Design review of the part built by this model. Coordinates are the model's own, in mm. Face numbers are marked on the shaded views. A direction names the side the tool comes from. Coordinates: 2 decimals unless noted, no trailing zeros. Loops run counter-clockwise (first coordinate to the right, second up) from the corner with the lowest first, then second, coordinate; pieces in that order, holes last. Notation, with made-up numbers: (73.25, -13) - (127.25, -13) arc R14 cw to (127.25, 9) - close; hole circle Ø7 at (6, 73). An arc over 180 degrees is marked (long way). Return JSON: item names as keys, results as strings. Group by question number.
from build123d import *

# Parameters (mm, degrees)
BOSS_EXTRUDE1_DEPTH         = 41.5925
SHELL1_START                = -39.0525
SHELL1_DEPTH                = 78.105
BOSS_EXTRUDE2_START         = 38.1
SKETCH3_R                   = 12.7
BOSS_EXTRUDE2_DEPTH         = 38.1
SKETCH4_R                   = 11.43
CUT_EXTRUDE1_DEPTH          = 132.301928586
F_1_4_20_TAPPED_HOLE1_D     = 5.1054
F_1_4_20_TAPPED_HOLE1_DEPTH = 2.54


# Read off the part's stored shape, not the designer's step: Shell1
with BuildPart() as part:
    # Sketch2 → Boss-Extrude1 (new, symmetric)
    with BuildSketch(Plane.XY):
        with BuildLine():
            Line((9.525, 8.400260413), (28.575, 41.395828297))
            Line((28.575, 41.395828297), (-28.575, 41.395828297))
            Line((-28.575, 41.395828297), (-9.525, 8.400260413))
            ThreePointArc((-9.525, 8.400260413), (0, -12.7), (9.525, 8.400260413))
        make_face()
    extrude(amount=BOSS_EXTRUDE1_DEPTH, both=True)

    # Shell1 outline → Shell1 (cut)
    with BuildSketch(Plane.XY.offset(SHELL1_START)):
        with BuildLine():
            ThreePointArc((-6.330300915, 7.946879282), (0, -10.16), (6.330300915, 7.946879282))
            Line((6.330300915, 7.946879282), (25.642060633, 41.395828297))
            Line((25.642060633, 41.395828297), (-25.642060633, 41.395828297))
            Line((-25.642060633, 41.395828297), (-6.330300915, 7.946879282))
        make_face()
    extrude(amount=SHELL1_DEPTH, mode=Mode.SUBTRACT)

    # Sketch3 → Boss-Extrude2 (add)
    with BuildSketch(Plane.XY.offset(41.5925).offset(BOSS_EXTRUDE2_START)):
        with Locations(Location((0, 0, 0), (0, 0, 138.590377891))):
            Circle(SKETCH3_R)
    extrude(amount=-BOSS_EXTRUDE2_DEPTH)

    # Sketch4 → Cut-Extrude1 (cut, through all)
    with BuildSketch(Plane.XY.offset(79.6925)):
        Circle(SKETCH4_R)
    extrude(amount=-CUT_EXTRUDE1_DEPTH, mode=Mode.SUBTRACT)

    # 1/4-20 Tapped Hole1
    with Locations(Plane(origin=(0, 0, -41.5925), x_dir=(1, 0, 0), z_dir=(0, 0, -1))):
        with Locations((0, -35.045828297)):
            Hole(F_1_4_20_TAPPED_HOLE1_D / 2, depth=F_1_4_20_TAPPED_HOLE1_DEPTH)


solid = part.part
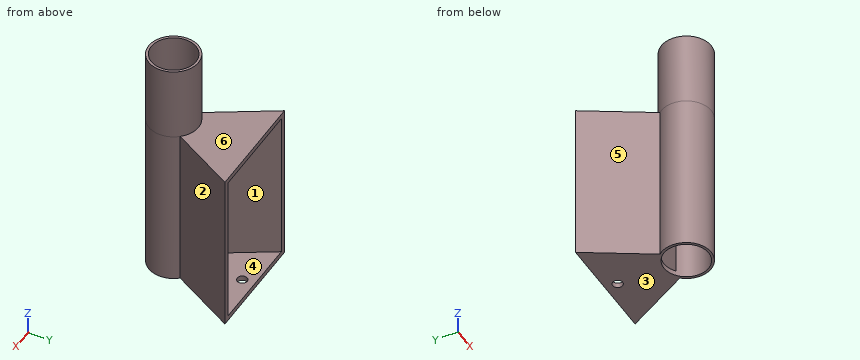
Item 1: Add section D-D (y = 20.5). State the section outline as (x, z) points, then the cut area to 3 significant figures.
Item 2: For the marked faces 1, 2 and 3, list the 3-axis set-ups (+Z, -Z, +X, -X, +Y, -Y) from which the entire face can be reached by the end or side of a thin tool; tool diameter is ignored.
Item 3: Add section A-A (x = 0). State the section outline as (y, z) points, then the cut area to 3 significant figures.
Item 4: Add section B-B (y = -3.5). State the section outline as (x, z) points.
Item 5: For P1, Ø6, axis at x = 0, y = 35.05, coming from the +Z side; P2, Ø12, axis at x = 11, z = 60, coming from the +Y side; P3, Ø10, axis at x = -15.5, z = 64.5, coming from the +Y side; P4, Ø18.5, axis at x = 0, y = 0, coming from the -Z side, all flat-tipped, find the tip position at first contact; note any pin that passes through.
Item 6: Add section C-C (z = 5). State the section outline as (x, y) points (3 decimals).
Item 7: Draft analysis for pull direction Z (two halves, no side actions). For the marked faces 4, 5 and 6, state which applies: pulls with the +Z half, pulls with the -Z half, needs draft (parallel to the pull), parting line crosses it, or undercut.
Item 8: To check wall thickness, follow line 1 (Z direction, x = -13, y = 36.5); line 2 (Y direction, x = 0, z = -40.3); line 3 (X direction, y = 12, z = 16). State the ranges of each line that lie inside material, in increasing order. Write a range as from..to.
Answers below:
{
 "1": {"outline": "(-16.51, -41.59) - (16.51, -41.59) - (16.51, 41.59) - (-16.51, 41.59) - close; hole (-13.58, -39.05) - (13.58, -39.05) - (13.58, 39.05) - (-13.58, 39.05) - close", "area": "626 mm^2"},
 "2": {"face 1": "+Y", "face 2": "+Z, -Z, +X", "face 3": "-Z, +X, -X, +Y, -Y"},
 "3": {"outline": "(-12.7, -41.59) - (-11.43, -41.59) - (-11.43, 79.69) - (-12.7, 79.69) - close; (11.43, -41.59) - (32.49, -41.59) - (32.49, -39.05) - (11.43, -39.05) - close; (11.43, 39.05) - (41.4, 39.05) - (41.4, 41.59) - (12.7, 41.59) - (12.7, 79.69) - (11.43, 79.69) - close; (37.6, -41.59) - (41.4, -41.59) - (41.4, -39.05) - (37.6, -39.05) - close", "area": "342 mm^2"},
 "4": {"outline": "(-12.21, -41.59) - (-10.88, -41.59) - (-10.88, 79.69) - (-12.21, 79.69) - close; (10.88, -41.59) - (12.21, -41.59) - (12.21, 79.69) - (10.88, 79.69) - close"},
 "5": {"P1": "stops at z = 41.59", "P2": "stops at y = 11.67", "P3": "stops at y = 7.14", "P4": "passes through"},
 "6": {"outline": "(-28.575, 41.396) - (-9.525, 8.4) arc R12.7 ccw (long way) to (9.525, 8.4) - (28.575, 41.396) - (25.642, 41.396) - (6.972, 9.058) arc R11.43 cw (long way) to (-6.972, 9.058) - (-25.642, 41.396) - close"},
 "7": {"face 4": "undercut", "face 5": "needs draft", "face 6": "pulls with the +Z half"},
 "8": {"line 1": "z = -41.59..-39.05, 39.05..41.59", "line 2": "y = -12.7..-11.43, 11.43..32.49, 37.6..41.4", "line 3": "x = -11.6..-8.67, 8.67..11.6"}
}
